Answer from the drawing. Dimensions are ordinates in mm from the lowest x, y and z of the part. A direction names the side the tool comes from. Coordinates: 2 decimals unless noted, no trailing zeros. Loops run counter-clockwise (first coordinate to the right, second up) from the corner with the lowest first, then second, coordinate; pieces in that order, holes last. Notation, with made-up numbers: (-10, -1.5) - (34, -1.5) arc R5 cw to (34, 6.5) - close; hole circle Ø4 at (11, -7). An arc over 180 degrees is marked (long way). Use one line per item in the form item = value. Start each with the question number.
1) A cutting plane is placed at A-A (y = 0.5). Give the vertices of the cut face in (x, z) (1 decimal), and give its area (3 significant figures).
2) A cutting plane is placed at B-B (z = 3.75). Give the vertices of the cut face in (x, y), and give its area (3 significant figures).
3) Each of these flat-tipped pins is pushed along its axis until it touches: P1, Ø3, axis at y = 5.5, z = 2.5, coming from the +X side; P2, Ø1.4, axis at y = 1, z = 1, coming from the -X side; P3, Ø2, axis at y = 4.5, z = 5, coming from the -X side. Where does it stop, or does it pass through?
4) Consider line 1 (X direction, y = 1.5, z = 0.5); line 2 (X direction, y = 0.5, z = 2.25); line 3 (Z direction, x = 17, y = 6.5) (1 decimal). Determine where each line is inside the solid, lowest interval first.
5) A cutting plane is placed at C-C (y = 5.75). Give the vertices of the cut face in (x, z) (1 decimal), and give its area (3 significant figures).
6) Which of the six approach directions +Z, -Z, +X, -X, +Y, -Y give full straight-line access (tool end or side, diameter ignored) to the marked faces 1, 2, 3, 4 and 5?
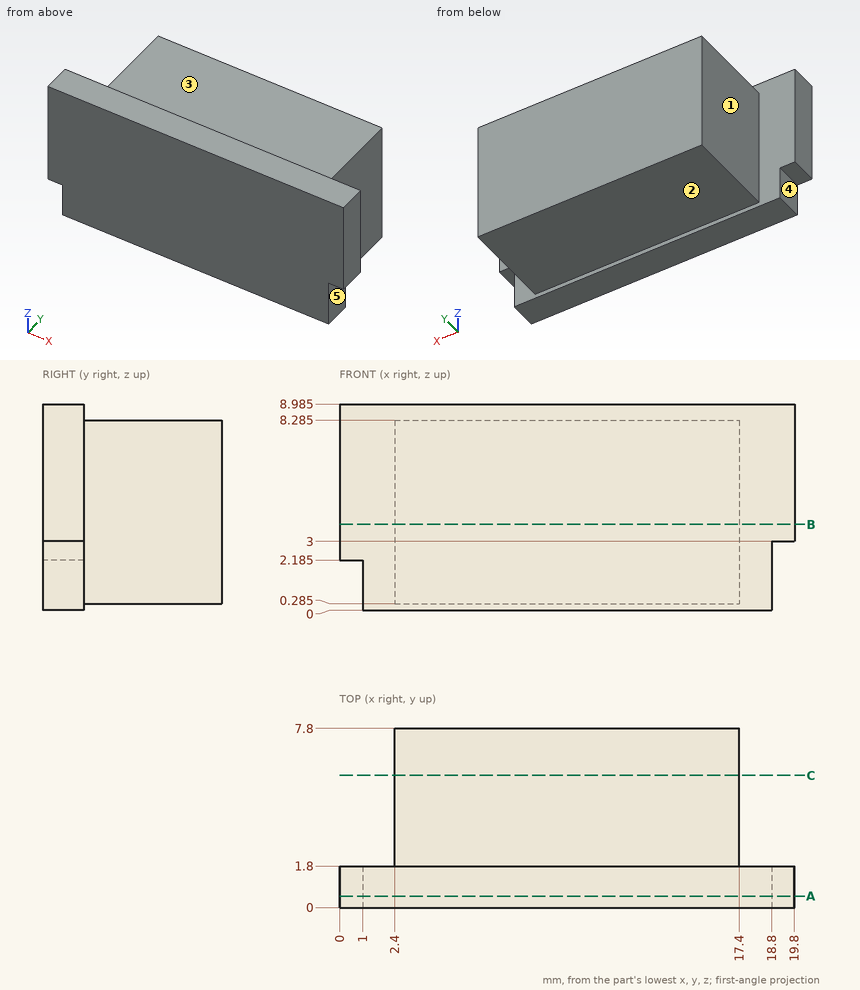
Found:
q1.outline = (0, 2.2) - (1, 2.2) - (1, 0) - (18.8, 0) - (18.8, 3) - (19.8, 3) - (19.8, 9) - (0, 9) - close
q1.area = 173 mm^2
q2.outline = (0, 0) - (19.8, 0) - (19.8, 1.8) - (17.4, 1.8) - (17.4, 7.8) - (2.4, 7.8) - (2.4, 1.8) - (0, 1.8) - close
q2.area = 126 mm^2
q3.P1 = 17.4
q3.P2 = 1
q3.P3 = 2.4
q4.line_1 = 1 to 18.8
q4.line_2 = 0 to 18.8
q4.line_3 = 0.3 to 8.3
q5.outline = (2.4, 0.3) - (17.4, 0.3) - (17.4, 8.3) - (2.4, 8.3) - close
q5.area = 120 mm^2
q6.face_1 = +Z, -Z, -X, +Y
q6.face_2 = -Z, +X, -X, +Y
q6.face_3 = +Z, +X, -X, +Y
q6.face_4 = -Z, -X, +Y, -Y
q6.face_5 = -Z, +X, +Y, -Y
